Part model, mm, in its own coordinate system. A direction names the side the tool comes from. Give positions to 0.01 mm unless a question says otherwise; leave off trailing zeros.
from build123d import *

# Parameters (mm, degrees)
BOSS_EXTRUDE1_DEPTH      = 20
FILLET1_R                = 60
FILLET2_R                = 10
CIRPATTERN1_COUNT        = 9
FILLET1_OF_CIRPATTERN1_R = 60
FILLET2_OF_CIRPATTERN1_R = 10


with BuildPart() as part:
    # Sketch1 → Revolve1 (revolve)
    with BuildSketch(Plane(origin=(0, 0, 0), x_dir=(0, 0, -1), z_dir=(1, 0, 0)), mode=Mode.PRIVATE) as revolve1_sk:
        Polygon((0, 0), (0, 100), (50, 100), (50, 417.5), (20, 417.5), (20, 462.5), (40, 462.5), (60.490381057, 457.009618943), (80, 437.5), (80, 0), align=None)
    revolve(revolve1_sk.sketch.rotate(Axis((0, 0, 404.979253112), (0, 0, -1)), 90), axis=Axis((0, 0, 404.979253112), (0, 0, -1)))

    # Sketch2 → Boss-Extrude1 (add)
    with BuildSketch(Plane.XY.offset(-50)):
        with BuildLine():
            Line((-20, 97.979589711), (-20, 417.02068294))
            ThreePointArc((-20, 417.02068294), (0, 417.5), (20, 417.02068294))
            Line((20, 417.02068294), (20, 97.979589711))
            ThreePointArc((20, 97.979589711), (0, 100), (-20, 97.979589711))
        make_face()
    boss_extrude1 = extrude(amount=BOSS_EXTRUDE1_DEPTH)

    # Fillet1
    fillet1_edges = [part.edges().sort_by_distance(p)[0] for p in [
        (-20, 417.02068294, -40),
    ]]
    fillet(fillet1_edges, radius=FILLET1_R)

    # Fillet2
    fillet2_edges = [part.edges().sort_by_distance(p)[0] for p in [
        (20, 417.02068294, -40),
        (20, 97.979589711, -40),
        (-20, 97.979589711, -40),
    ]]
    fillet(fillet2_edges, radius=FILLET2_R)

    # CirPattern1: Boss-Extrude1 ×9 about axis
    cirpattern1_axis = Axis((0, 0, 0), (0, 0, 1))
    for i in range(1, CIRPATTERN1_COUNT):
        add(boss_extrude1.rotate(cirpattern1_axis, i * 360 / CIRPATTERN1_COUNT))

    # Fillet1 of CirPattern1
    fillet1_of_cirpattern1_edges = [part.edges().sort_by_distance(p)[0] for p in [
        (-283.376616839, 306.600624638, -40),
        (-414.158165279, 52.718726582, -40),
        (-351.15050533, -225.830849546, -40),
        (-123.835621333, -398.711661341, -40),
        (161.423326165, -385.030855608, -40),
        (371.15050533, -191.189833394, -40),
        (407.212238173, 92.111036702, -40),
        (252.734839115, 332.312129026, -40),
    ]]
    fillet(fillet1_of_cirpattern1_edges, radius=FILLET1_OF_CIRPATTERN1_R)

    # Fillet2 of CirPattern1
    fillet2_of_cirpattern1_edges = [part.edges().sort_by_distance(p)[0] for p in [
        (-252.734839115, 332.312129026, -40),
        (-47.659177406, 87.912472431, -40),
        (-78.300955131, 62.200968044, -40),
        (-407.212238173, 92.111036702, -40),
        (-93.018096031, 36.710132262, -40),
        (-99.964023138, -2.682177858, -40),
        (-371.15050533, -191.189833394, -40),
        (-94.852813742, -31.66928678, -40),
        (-74.852813742, -66.310302931, -40),
        (-161.423326165, -385.030855608, -40),
        (-52.304845732, -85.230294573, -40),
        (-14.7171409, -98.911100306, -40),
        (123.835621333, -398.711661341, -40),
        (14.7171409, -98.911100306, -40),
        (52.304845732, -85.230294573, -40),
        (351.15050533, -225.830849546, -40),
        (74.852813742, -66.310302931, -40),
        (94.852813742, -31.66928678, -40),
        (414.158165279, 52.718726582, -40),
        (99.964023138, -2.682177858, -40),
        (93.018096031, 36.710132262, -40),
        (283.376616839, 306.600624638, -40),
        (78.300955131, 62.200968044, -40),
        (47.659177406, 87.912472431, -40),
    ]]
    fillet(fillet2_of_cirpattern1_edges, radius=FILLET2_OF_CIRPATTERN1_R)


solid = part.part
1) Drill centre lines: L1, parallel to Y at x = 0, z = -28; L2, parallel to Y at x = 0, z = -39; L3, parallel to Z at x = 395, y = -99. Where is each one in solid material? Low to high.
Check result:
L1: y = -462.5 to -417.5, -100 to 100, 417.5 to 462.5
L2: y = -462.5 to -417.5, -100 to 462.5
L3: z = -80 to -50
2) 3-axis set-ups, long thin cutter, end or side, ignore diameter. For faces 1 (the flat face through (1, -1, 0)), 2 (the flat face through (266, 46, -30)): which of +Z, -Z, +X, -X, +Y, -Y reach the whole face in a straight line?
Check result:
face 1: +Z, +X, -X, +Y, -Y
face 2: +Z
3) Flat gauge pins, fed straight in: P1, Ø1.5, axis at x = -249, y = -3, coming from the +Z side; P2, Ø6, axis at y = 22, z = -14, coming from the -X side; P3, Ø12, axis at y = -323.5, z = -52, coming from the +X side. Where does each tip first touch, or does it go through?
Check result:
P1: stops at z = -50
P2: stops at x = -98.18
P3: stops at x = 332.28
